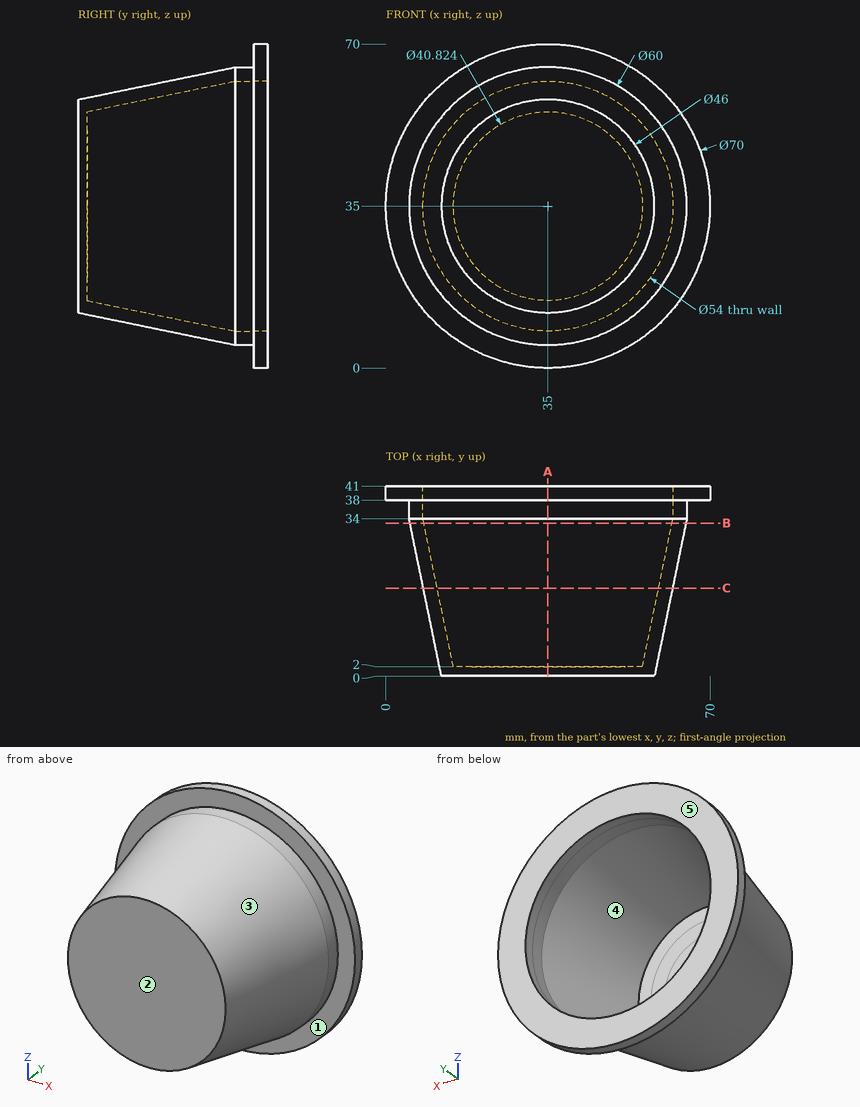
For this review, use the dimensioned drawing (mm, ordinates from the lowest corner) and the shaded views. A direction names the side the tool comes from. Give positions to 0.01 mm unless a question says otherwise; leave off trailing zeros. Write each loop counter-clockwise with the first axis right and the second up, starting at its lowest first coordinate (ties: lowest second). Pieces come first, ordered by that corner, then holes.
(1) Consider section B-B, the plane y = 33. Give the boundary of the cut face in (x, z) (1 decimal).
(2) Consider section C-C, the plane y = 19. Give the boundary of the cut face in (x, z).
(3) The part is to be moulded in two halves that separate along Z. For the marked faces 3, 4 and 5, say which applies: released by +Z, released by -Z, zero draft, split by the parting line, or undercut.
(4) Consider section A-A, the plane x = 35. Give the boundary of the cut face in (y, z), and give its area (3 significant figures).
(5) To check wall thickness, follow L1, parallel to Z at x = 35, y = 36.55; L2, parallel to Y at x = 37, z = 29; L3, parallel to Z at x = 35, y = 38.75. State the ranges of each line that lie inside material, in increasing order.
(6) For P1, Ø10, axis at x = 32, y = 10, coming from the -Z side; P2, Ø20.5, axis at x = 29.5, z = 39.5, coming from the +Y side; P3, Ø12, axis at y = 34.5, z = 15, coming from the +X side, all flat-tipped, find the tip position at first contact; note any pin that passes through.
(7) Tool access review of the marked faces 1 and 2: name each direction out of +Z, -Z, +X, -X, +Y, -Y from which nothing blocks a thin tool from reaching the whole face with its end or side.
Returned:
1. outline: circle Ø59.6 at (35, 35); hole circle Ø53.6 at (35, 35)
2. outline: circle Ø53.82 at (35, 35); hole circle Ø47.82 at (35, 35)
3. face 3: split by the parting line
3. face 4: undercut
3. face 5: zero draft
4. outline: (0, 12) - (34, 5) - (38, 5) - (38, 0) - (41, 0) - (41, 8) - (34, 8) - (2, 14.59) - (2, 55.41) - (34, 62) - (41, 62) - (41, 70) - (38, 70) - (38, 65) - (34, 65) - (0, 58) - close
4. area: 357 mm2
5. L1: z = 5 to 8, 62 to 65
5. L2: y = 0 to 2
5. L3: z = 0 to 8, 62 to 70
6. P1: stops at z = 9
6. P2: stops at y = 2
6. P3: stops at x = 66.56
7. face 1: -Y
7. face 2: +Z, -Z, +X, -X, -Y
